from build123d import *

# Parameters (mm, degrees)
F1_DEPTH = 20
F2_R     = 3
F3_R     = 21.3660555905
F4_R     = 4
F7_DEPTH = 6.7
F7_TAPER = 1.25
F8_D     = 5.5
F8_DEPTH = 2
F8_START = 6.7
F8_TIP   = 1.6523667023
F9_R     = 2


with BuildPart() as f1:
    # F0 (on Front) → F1 (new body)
    with BuildSketch(Plane.XZ):
        with BuildLine():
            Line((-25, -25), (25, -25))
            Line((25, -25), (25, 25))
            Line((25, 25), (12.5, 25))
            Line((12.5, 25), (12.5, 0))
            ThreePointArc((12.5, 0), (0, -12.5), (-12.5, 0))
            Line((-12.5, 0), (-12.5, 25))
            Line((-12.5, 25), (-25, 25))
            Line((-25, 25), (-25, -25))
        make_face()
    extrude(amount=F1_DEPTH)

    # F2
    f2_edges = [f1.edges().sort_by_distance(p)[0] for p in [
        (12.5, -10, 25),
        (-12.5, -10, 25),
        (-25, -10, 25),
    ]]
    fillet(f2_edges, radius=F2_R)

    # F3
    f3_edges = [f1.edges().sort_by_distance(p)[0] for p in [
        (-25, -10, -25),
    ]]
    fillet(f3_edges, radius=F3_R)

    # F4 (on face) → F7 (cut)
    with BuildSketch(Plane.YZ.offset(25)):
        with Locations((-10, 16)):
            Circle(F4_R)
        with Locations((-10, -16)):
            Circle(F4_R)
    extrude(amount=-F7_DEPTH, taper=F7_TAPER, mode=Mode.SUBTRACT)

    # F8
    # its depths count from where the whole tool has entered the part; down to there all is cleared
    with Locations(Plane.YZ.offset(25)):
        with Locations((-10, 16), (-10, -16)):
            Hole(F8_D / 2, depth=F8_START)
    with Locations(Plane.YZ.offset(25).offset(-F8_START)):
        with Locations((-10, 16), (-10, -16)):
            Hole(F8_D / 2, depth=F8_DEPTH)
            with Locations((0, 0, -(F8_DEPTH + F8_TIP / 2))):  # 118° drill point
                Cone(0, F8_D / 2, F8_TIP, mode=Mode.SUBTRACT)

    # F9
    f9_edges = [f1.edges().sort_by_distance(p)[0] for p in [
        (20.25, 0, 25),
        (20.25, -20, 25),
    ]]
    fillet(f9_edges, radius=F9_R)


solid = f1.part
Read the model definition and answer for the solid it produces. Units are mm, in the model's axes. A direction names the side the tool comes from. Coordinates: 2 decimals unless noted, no trailing zeros. Order: outer loops, then holes, each group sorted by start corner. A loop starts at its lowest first (then second) coordinate and runs counter-clockwise, first axis right, second up. Notation, with made-up numbers: (23, 4.25) -> (61, 4.25) arc R11 ccw to (61, 13.25) -> close; hole circle Ø1 at (-20, 65). An arc over 180 degrees is marked (long way). Answer as a JSON object with one key per item and string values.
1) Consider line 1 along Z through (x, y) = (17.8, -10); line 2 along X through (y, z) = (-8, 5); line 3 along Y through (x, z) = (17.15, -16). Determine where each line is inside the solid, lowest interval first. Write a range as from..to.
Model answer:
{"line 1": "z = -25..-18.75, -13.25..13.25, 18.75..25", "line 2": "x = -25..-12.5, 12.5..25", "line 3": "y = -20..-12.75, -7.25..0"}
2) A cutting plane is placed at B-B, the plane y = -5. Determine the outline of the cut face in (x, z).
Model answer:
{"outline": "(-25, -3.63) arc R21.37 ccw to (-3.63, -25) -> (25, -25) -> (25, 25) -> (15.5, 25) arc R3 ccw to (12.5, 22) -> (12.5, 0) arc R12.5 cw to (-12.5, 0) -> (-12.5, 22) arc R3 ccw to (-15.5, 25) -> (-22, 25) arc R3 ccw to (-25, 22) -> close"}
3) Each of these flat-tipped pins is pushed along its axis until it touches: pin 1 (2.5 mm diameter, centred on y = -12, z = 15.5, fed in from +X); pin 2 (2.5 mm diameter, centred on y = -10, z = -15.5, fed in from +X); pin 3 (1.5 mm diameter, centred on x = -4.5, y = -5.5, fed in from +Z). Where does it stop, or does it pass through?
Model answer:
{"pin 1": "stops at x = 18.3", "pin 2": "stops at x = 15.7", "pin 3": "stops at z = -11.34"}
4) A cutting plane is placed at A-A, the plane z = 3. Determine the outline of the cut face in (x, y), plus the area to 3 significant figures.
Model answer:
{"outline": "(-25, -18) arc R2 ccw to (-23, -20) -> (-14.5, -20) arc R2 ccw to (-12.5, -18) -> (-12.5, -2) arc R2 ccw to (-14.5, 0) -> (-23, 0) arc R2 ccw to (-25, -2) -> close; (12.5, -18) arc R2 ccw to (14.5, -20) -> (25, -20) -> (25, 0) -> (14.5, 0) arc R2 ccw to (12.5, -2) -> close", "area": "495 mm²"}
5) The mould has two halves that part along X. Classify faces 6 (the face through (-25, -10, 9)), 7 (the face through (20.18, -0.57, 24.4)), 8 (the face through (0.275, -9.888, -12.497)): released by +X, released by -X, zero draft, split by the parting line, or undercut.
Model answer:
{"face 6": "released by -X", "face 7": "zero draft", "face 8": "undercut"}
6) A tool of negligible diameter and unlimited length cuts with its end or side. For faces 1 (the face through (21.603, -6.255, -14.821)), 2 (the face through (-13.07, -19.4, 11.15)), 3 (the face through (11, 0, -10)), 4 (the face through (-13.36, -10.11, 24.1)), 5 (the face through (11, -20, -10)), from which of +Z, -Z, +X, -X, +Y, -Y can it reach the whole face along a straight path? Write none if from no direction.
Model answer:
{"face 1": "+X", "face 2": "+Z, -Y", "face 3": "+Z, -Z, +X, -X, +Y", "face 4": "+Z, +Y, -Y", "face 5": "+Z, -Z, +X, -X, -Y"}
